Autodesk Inventor part; units mm, degrees
ref_plane "YZ Plane" through (0, 0, 0) normal (1, 0, 0) x (0, 1, 0)
ref_plane "XZ Plane" through (0, 0, 0) normal (0, 1, 0) x (-1, 0, 0)
ref_plane "XY Plane" through (0, 0, 0) normal (0, 0, 1) x (1, 0, 0)
sketch "Sketch1" plane through (0, 0, 0) normal (0, 1, 0) x (-1, 0, 0)
  line L0 (-120, 120) -> (120, 120)
  line L1 (120, 120) -> (120, -120)
  line L2 (120, -120) -> (-120, -120)
  line L3 (-120, -120) -> (-120, 120)
  line L4 (-120, 120) -> (120, -120) construction
  line L5 (120, 120) -> (-120, -120) construction
  circle A0 centre (23.5, 29) radius 2.75
  circle A1 centre (23.5, -29) radius 2.75
  circle A2 centre (-23.5, 29) radius 2.75
  circle A3 centre (-23.5, -29) radius 2.75
  point P0 (0, 0)
  dimension "d0" = 240
  dimension "d1" = 240
  dimension "d4" = 5.5
  dimension "d7" = 58
  dimension "d10" = 47
  dimension "d13" = 29
  dimension "d14" = 29
  dimension "d15" = 23.5
  dimension "d16" = 23.5
extrude "Extrusion1" add sketch "Sketch1" along normal blind 12
properties part number "MDFTop"
Can you work these out from the model? Positions are in its coordinate system, mm. Round coordinates to 2 decimals unless told otherwise and drop trailing zeros. Loops run counter-clockwise (first coordinate to the right, second up) from the corner with the lowest first, then second, coordinate; pieces in that order, holes last.
Item 1: If we mould it in two halves opening along Z, with no side actions, what happens to faces 1 (the flat face through (2, 6, 120)), 2 (the flat face through (120, 6, -2)), 3 (the cylindrical face through (26.247, 5.916, -29.121)), 4 (the flat face through (-2, 6, -120))? For each: +Z half, -Z half, draft (parallel to the pull), parting line (faces both ways), or undercut.
Item 2: Please list where this line runs through material, in increasing order: L1, parallel to Z at x = -23.5, y = 3.
Item 3: Suppose I cut it at A-A, the plane z = -29. Write out the boundary of the cut face in (x, y), then the cut area to 3 significant figures.
Item 4: Will this pin go through, and if not, where does the flat tip stop? pin 1 Ø7 at (x, z) = (23.5, -29) entering from -Y.
Item 5: Suppose I cut it at B-B, the plane x = -23.5. Write out the boundary of the cut face in (y, z).
Reported:
1. face 1: +Z half
1. face 2: draft
1. face 3: undercut
1. face 4: -Z half
2. L1: z = -120 to -31.75, -26.25 to 26.25, 31.75 to 120
3. outline: (-120, 0) - (-26.25, 0) - (-26.25, 12) - (-120, 12) - close; (-20.75, 0) - (20.75, 0) - (20.75, 12) - (-20.75, 12) - close; (26.25, 0) - (120, 0) - (120, 12) - (26.25, 12) - close
3. area: 2,750 mm2
4. pin 1: stops at y = 0
5. outline: (0, -120) - (12, -120) - (12, -31.75) - (0, -31.75) - close; (0, -26.25) - (12, -26.25) - (12, 26.25) - (0, 26.25) - close; (0, 31.75) - (12, 31.75) - (12, 120) - (0, 120) - close
